Here's how the part is built. I have some questions about the finished solid (model axes, mm). Coordinates: 2 decimals unless noted, no trailing zeros. Write each loop counter-clockwise with the first axis right and the second up, starting at its lowest first coordinate (ties: lowest second). Pieces come first, ordered by that corner, then holes.
(1) Imagine slicing it at B-B, the plane z = 15. List the corners of the cut face in (x, y) for me, plus the area to 3 significant figures.
(2) Imagine slicing it at C-C, the plane x = 6. List the corners of the cut face in (y, z) for me.
(3) For pin 1 Ø1.5 at (x, z) = (16, 1) entering from +Y; pin 2 Ø1.5 at (y, z) = (0.5, -14.5) entering from -X; pin 3 Ø2.5 at (y, z) = (1.5, -14.5) entering from +X; pin 4 Ø2.5 at (x, y) = (4, 2) entering from -Z, each with a flat end and sliding along its axis, tell me the tip position at first contact or that it passes through.
(4) Imagine slicing it at A-A, the plane x = 20. List the corners of the cut face in (y, z) for me.
(5) Imagine slicing it at D-D, the plane z = -15. List the corners of the cut face in (x, y) for me.
(6) Please list where these lines run through material, in increasing order: probe 1 along Z at (x, y) = (20, -0.45); probe 2 along X at (y, z) = (-0.75, 15); probe 3 along Y at (x, z) = (11, 13).
```python
from build123d import *

# Parameters (mm, degrees)
SKETCH_1_W          = 47
SKETCH_1_H          = 37
EXTRUDE_1_DEPTH     = 1.6
SKETCH_2_R          = 1.3
CUT_EXTRUDE_1_DEPTH = 1.6
SKETCH_3_W          = 32
SKETCH_3_H          = 5
EXTRUDE_2_DEPTH     = 3


with BuildPart() as part:
    # Эскиз1 → Бобышка-Вытянуть1 (new body)
    with BuildSketch(Plane(origin=(0, 0, 0), x_dir=(1, 0, 0), z_dir=(0, 1, 0))):
        Rectangle(SKETCH_1_W, SKETCH_1_H)
    extrude(amount=-EXTRUDE_1_DEPTH)

    # Эскиз2 → Вырез-Вытянуть1 (cut)
    with BuildSketch(Plane(origin=(0, 0, 0), x_dir=(1, 0, 0), z_dir=(0, 1, 0))):
        with Locations((-20, 15)):
            Circle(SKETCH_2_R)
        with Locations((-20, -15)):
            Circle(SKETCH_2_R)
        with Locations((20, -15)):
            Circle(SKETCH_2_R)
        with Locations((20, 15)):
            Circle(SKETCH_2_R)
    extrude(amount=-CUT_EXTRUDE_1_DEPTH, mode=Mode.SUBTRACT)

    # Эскиз3 → Бобышка-Вытянуть2 (add)
    with BuildSketch(Plane(origin=(0, 0, 0), x_dir=(1, 0, 0), z_dir=(0, 1, 0))):
        with Locations((0, 15)):
            Rectangle(SKETCH_3_W, SKETCH_3_H)
    extrude(amount=EXTRUDE_2_DEPTH)


solid = part.part
```
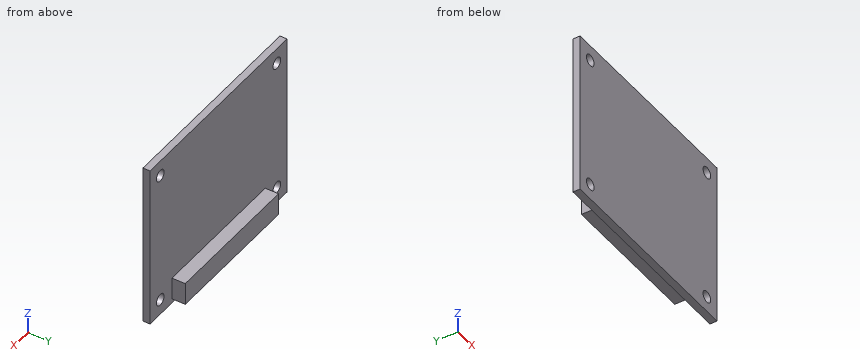
Recorded:
1. outline: (-23.5, -1.6) - (-21.3, -1.6) - (-21.3, 0) - (-23.5, 0) - close; (-18.7, -1.6) - (18.7, -1.6) - (18.7, 0) - (-18.7, 0) - close; (21.3, -1.6) - (23.5, -1.6) - (23.5, 0) - (21.3, 0) - close
1. area: 66.9 mm2
2. outline: (-1.6, -18.5) - (0, -18.5) - (0, -17.5) - (3, -17.5) - (3, -12.5) - (0, -12.5) - (0, 18.5) - (-1.6, 18.5) - close
3. pin 1: stops at y = 0
3. pin 2: stops at x = -23.5
3. pin 3: stops at x = 16
3. pin 4: stops at z = -17.5
4. outline: (-1.6, -18.5) - (0, -18.5) - (0, -16.3) - (-1.6, -16.3) - close; (-1.6, -13.7) - (0, -13.7) - (0, 13.7) - (-1.6, 13.7) - close; (-1.6, 16.3) - (0, 16.3) - (0, 18.5) - (-1.6, 18.5) - close
5. outline: (-23.5, -1.6) - (-21.3, -1.6) - (-21.3, 0) - (-23.5, 0) - close; (-18.7, -1.6) - (18.7, -1.6) - (18.7, 0) - (16, 0) - (16, 3) - (-16, 3) - (-16, 0) - (-18.7, 0) - close; (21.3, -1.6) - (23.5, -1.6) - (23.5, 0) - (21.3, 0) - close
6. probe 1: z = -18.5 to -16.3, -13.7 to 13.7, 16.3 to 18.5
6. probe 2: x = -23.5 to -21.3, -18.7 to 18.7, 21.3 to 23.5
6. probe 3: y = -1.6 to 0
